Geometry: final body of the model. Coordinates: model frame, mm. A direction names the side the tool comes from. Give positions to 0.01 mm unless a question says otherwise; leave off trailing zeros. Loops run counter-clockwise (first coordinate to the right, second up) from the corner with the lowest first, then second, coordinate; pieces in that order, holes last.
1. Section C-C, the plane y = 0. Output: boundary loops of the cut face in (x, z).
2. Draft query along Z for faces 1 (the face through (-25.4, 63, 116)), 2 (the face through (-4, -152.4, 38)), 3 (the face through (-5, 2, 0)). Return one class per face: +Z half, -Z half, draft (parallel to the pull), parting line (faces both ways), or undercut.
3. Material intervals for line 1 along Y through (x, z) = (-177, 49); line 2 along X through (y, z) = (-110, 269); line 3 along Z through (x, y) = (127, 43.5), sorted ascending.
4. Section D-D, the plane z = 327. Output: boundary loops of the cut face in (x, y).
5. Section A-A, the plane x = 0. Output: boundary loops of the cut face in (y, z).
6. First-contact query: P1, Ø8, axis at y = 15, z = 118, coming from the -X side; P2, Ø12, axis at x = 198.5, y = -6.5, coming from the +Z side; P3, Ø15, axis at y = 9.5, z = 160, coming from the +X side; P4, Ø4, axis at x = -59.5, y = -96.5, coming from the -Z side. Flat tips, straight axial feed; report the tip coordinate or a pass-through.
7. Access query for faces 4 (the face through (63, -25.4, 131)), 5 (the face through (-64, 25.4, 131)), 6 (the face through (101.6, 0, 144)). Directions: +Z, -Z, +X, -X, +Y, -Y. A direction counts if a zero-diameter tool reaches every point of the face in a straight line with its end or side. Return the directions, or none.
8. Section B-B, the plane z = 198.5. Output: boundary loops of the cut face in (x, y), then the cut area to 3 significant figures.
from build123d import *

# Parameters (mm, degrees)
F0_R     = 38.1
F0_W     = 228.6
F0_H     = 304.8
F0_R_2   = 22.225
F1_DEPTH = 76.2
F2_SIZE2 = 10.998523
F2_SIZE  = 6.35
F4_DEPTH = 101.6
F5_DEPTH = 25.4
F3_R     = 76.2
F6_DEPTH = 152.4


with BuildPart() as f1:
    # F0 (on Top) → F1 (new body)
    with BuildSketch(Plane.XY):
        with BuildLine():
            Line((-114.3, 152.4), (-304.8, 152.4))
            ThreePointArc((-304.8, 152.4), (-358.681537, 130.081537), (-381, 76.2))
            Line((-381, 76.2), (-304.8, 76.2))
            ThreePointArc((-304.8, 76.2), (-228.6, 0), (-304.8, -76.2))
            Line((-304.8, -76.2), (-381, -76.2))
            ThreePointArc((-381, -76.2), (-358.681537, -130.081537), (-304.8, -152.4))
            Line((-304.8, -152.4), (-114.3, -152.4))
            Line((-114.3, -152.4), (-114.3, 152.4))
        make_face()
        with Locations((-177.8, -76.2)):
            Circle(F0_R, mode=Mode.SUBTRACT)
        with Locations((-177.8, 76.2)):
            Circle(F0_R, mode=Mode.SUBTRACT)
        Rectangle(F0_W, F0_H)
        with BuildLine():
            Line((304.8, 152.4), (114.3, 152.4))
            Line((114.3, 152.4), (114.3, -152.4))
            Line((114.3, -152.4), (304.8, -152.4))
            ThreePointArc((304.8, -152.4), (358.681537, -130.081537), (381, -76.2))
            Line((381, -76.2), (304.8, -76.2))
            ThreePointArc((304.8, -76.2), (228.6, 0), (304.8, 76.2))
            Line((304.8, 76.2), (381, 76.2))
            ThreePointArc((381, 76.2), (358.681537, 130.081537), (304.8, 152.4))
        make_face()
        with Locations((177.8, -76.2)):
            Circle(F0_R, mode=Mode.SUBTRACT)
        with Locations((177.8, 76.2)):
            Circle(F0_R, mode=Mode.SUBTRACT)
        with Locations((177.8, 76.2)):
            Circle(F0_R)
        with Locations((177.8, 76.2)):
            Circle(F0_R_2, mode=Mode.SUBTRACT)
        with Locations((177.8, -76.2)):
            Circle(F0_R)
        with Locations((177.8, -76.2)):
            Circle(F0_R_2, mode=Mode.SUBTRACT)
        with Locations((-177.8, -76.2)):
            Circle(F0_R)
        with Locations((-177.8, -76.2)):
            Circle(F0_R_2, mode=Mode.SUBTRACT)
        with Locations((-177.8, 76.2)):
            Circle(F0_R)
        with Locations((-177.8, 76.2)):
            Circle(F0_R_2, mode=Mode.SUBTRACT)
    extrude(amount=F1_DEPTH)

    # F2
    f2_edges = [f1.edges().sort_by_distance(p)[0] for p in [
        (-200.025, 76.2, 76.2),
        (-200.025, -76.2, 76.2),
        (155.575, -76.2, 76.2),
        (155.575, 76.2, 76.2),
    ]]
    chamfer(f2_edges, length=F2_SIZE, length2=F2_SIZE2)

    # F3 (on Front) → F4 (join, symmetric)
    with BuildSketch(Plane.XZ):
        with BuildLine():
            ThreePointArc((25.4, 155.257952), (0, 152.4), (-25.4, 155.257952))
            Line((-25.4, 155.257952), (-25.4, 76.2))
            Line((-25.4, 76.2), (25.4, 76.2))
            Line((25.4, 76.2), (25.4, 155.257952))
        make_face()
    extrude(amount=F4_DEPTH, both=True)

    # F3 (on Front) → F5 (join, symmetric)
    with BuildSketch(Plane.XZ):
        with BuildLine():
            Line((101.6, 76.2), (101.6, 214.336559))
            ThreePointArc((101.6, 214.336559), (70.034423, 176.369111), (25.4, 155.257952))
            Line((25.4, 155.257952), (25.4, 76.2))
            Line((25.4, 76.2), (101.6, 76.2))
        make_face()
        with BuildLine():
            ThreePointArc((-25.4, 155.257952), (-70.034423, 176.369111), (-101.6, 214.336559))
            Line((-101.6, 214.336559), (-101.6, 76.2))
            Line((-101.6, 76.2), (-25.4, 76.2))
            Line((-25.4, 76.2), (-25.4, 155.257952))
        make_face()
    extrude(amount=F5_DEPTH, both=True)

    # F3 (on Front) → F6 (join, symmetric)
    with BuildSketch(Plane.XZ):
        with BuildLine():
            ThreePointArc((101.6, 214.336559), (111.079634, 239.759232), (114.3, 266.7))
            ThreePointArc((114.3, 266.7), (-26.940768, 377.779634), (-101.6, 214.336559))
            ThreePointArc((-101.6, 214.336559), (-70.034423, 176.369111), (-25.4, 155.257952))
            ThreePointArc((-25.4, 155.257952), (0, 152.4), (25.4, 155.257952))
            ThreePointArc((25.4, 155.257952), (70.034423, 176.369111), (101.6, 214.336559))
        make_face()
        with Locations((0, 266.7)):
            Circle(F3_R, mode=Mode.SUBTRACT)
    extrude(amount=F6_DEPTH, both=True)


solid = f1.part
Answers below:
1. outline: (-228.6, 0) - (228.6, 0) - (228.6, 76.2) - (101.6, 76.2) - (101.6, 214.34) arc R114.3 ccw to (114.3, 266.7) arc R114.3 ccw (long way) to (-101.6, 214.34) - (-101.6, 76.2) - (-228.6, 76.2) - close; hole circle Ø152.4 at (0, 266.7)
2. face 1: undercut
2. face 2: draft
2. face 3: -Z half
3. line 1: y = -152.4 to -98.41, -53.99 to 53.99, 98.41 to 152.4
3. line 2: x = -114.28 to -76.17, 76.17 to 114.28
3. line 3: z = 0 to 76.2
4. outline: (-97.1, -152.4) - (-46.59, -152.4) - (-46.59, 152.4) - (-97.1, 152.4) - close; (46.59, -152.4) - (97.1, -152.4) - (97.1, 152.4) - (46.59, 152.4) - close
5. outline: (-152.4, 0) - (152.4, 0) - (152.4, 76.2) - (101.6, 76.2) - (101.6, 152.4) - (152.4, 152.4) - (152.4, 190.5) - (-152.4, 190.5) - (-152.4, 152.4) - (-101.6, 152.4) - (-101.6, 76.2) - (-152.4, 76.2) - close; (-152.4, 342.9) - (152.4, 342.9) - (152.4, 381) - (-152.4, 381) - close
6. P1: stops at x = -101.6
6. P2: stops at z = 76.2
6. P3: stops at x = 101.6
6. P4: stops at z = 0
7. face 4: +X, -Y
7. face 5: -X, +Y
7. face 6: +X, +Y, -Y
8. outline: (-101.6, -25.4) - (-91.72, -25.4) - (-91.72, -152.4) - (-33.99, -152.4) - (-33.99, 152.4) - (-91.72, 152.4) - (-91.72, 25.4) - (-101.6, 25.4) - close; (33.99, -152.4) - (91.72, -152.4) - (91.72, -25.4) - (101.6, -25.4) - (101.6, 25.4) - (91.72, 25.4) - (91.72, 152.4) - (33.99, 152.4) - close
8. area: 36,200 mm2
